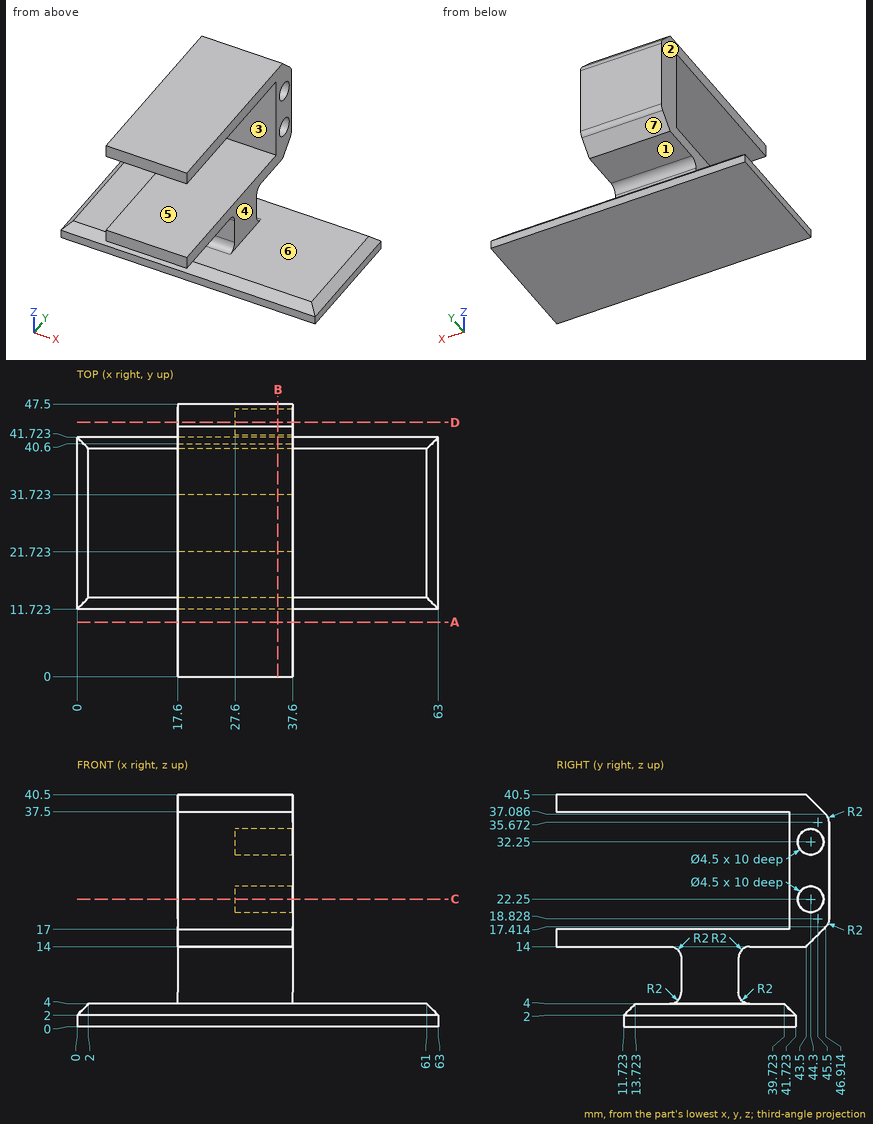
For this review, use the dimensioned drawing (mm, ordinates from the lowest corner) and the shaded views. A direction names the side the tool comes from. Give positions to 0.01 mm unless a question says otherwise; leave off trailing zeros. Write each loop counter-clockwise with the first axis right and the second up, starting at its lowest first coordinate (ties: lowest second). Pieces come first, ordered by that corner, then holes.
(1) The part is to be moulded in two halves that separate along Z. For the marked faces 4, 5, 6 and 7, say which applies: released by +Z, released by -Z, zero draft, split by the parting line, or undercut.
(2) Consider section C-C, the plane z = 22.25. Give the boundary of the cut face in (x, y).
(3) To check wall thickness, follow L1, parallel to Z at x = 31, y = 44; L2, parallel to Y at x = 30.25, z = 22.25; L3, parallel to Z at x = 24.5, y = 31.5. State the ranges of each line that lie inside material, in increasing order.
(4) For P1, Ø5, axis at x = 31.5, z = 10, coming from the -Y side; P2, Ø2, axis at y = 44, z = 21.5, coming from the +X side; P3, Ø3, axis at x = 29.5, z = 10.5, coming from the +Y side; P4, Ø10, axis at x = 17, y = 42, coming from the +Z side, all flat-tipped, find the tip position at first contact; note any pin that passes through.
(5) Tool access review of the marked faces 1, 2 and 3: name each direction out of +Z, -Z, +X, -X, +Y, -Y from which nothing blocks a thin tool from reaching the whole face with its end or side.
(6) Consider section D-D, the plane y = 44.3. Give the boundary of the cut face in (x, z).
(7) Consider section B-B, the plane x = 35. Give the number of separate pieces and of enclosed holes in the cut face, and give its area (3 significant figures).
(8) Consider section A-A, the plane y = 9.5. Give the boundary of the cut face in (x, z), and give its area (3 significant figures).
Returned:
1. face 4: zero draft
1. face 5: undercut
1. face 6: undercut
1. face 7: released by -Z
2. outline: (17.6, 40.6) - (37.6, 40.6) - (37.6, 42.05) - (27.6, 42.05) - (27.6, 46.55) - (37.6, 46.55) - (37.6, 47.5) - (17.6, 47.5) - close
3. L1: z = 14.5 to 20.02, 24.48 to 30.02, 34.48 to 40
3. L2: y = 40.6 to 42.05, 46.55 to 47.5
3. L3: z = 0 to 17, 37.5 to 40.5
4. P1: stops at y = 21.66
4. P2: stops at x = 27.6
4. P3: stops at y = 31.72
4. P4: stops at z = 40.5
5. face 1: +X, -X, +Y
5. face 2: +Z, -X, +Y, -Y
5. face 3: +X, -X, -Y
6. outline: (17.6, 14.8) - (37.6, 14.8) - (37.6, 20) - (27.6, 20) - (27.6, 24.5) - (37.6, 24.5) - (37.6, 30) - (27.6, 30) - (27.6, 34.5) - (37.6, 34.5) - (37.6, 39.7) - (17.6, 39.7) - close
7. separate pieces: 1
7. enclosed holes: 2
7. area: 598 mm2
8. outline: (17.6, 14) - (37.6, 14) - (37.6, 17) - (17.6, 17) - close; (17.6, 37.5) - (37.6, 37.5) - (37.6, 40.5) - (17.6, 40.5) - close
8. area: 120 mm2
